Geometry: final body of the model. Coordinates: model frame, mm. Face numbers are marked on the shaded views. A direction names the side the tool comes from. Give positions to 0.01 mm unless a question says otherwise; leave off trailing zeros. Loops run counter-clockwise (first coordinate to the right, second up) from the corner with the lowest first, then second, coordinate; pieces in that order, holes last. Notation, with made-up numbers: (36.25, -30.75) -> (41.25, -30.75) arc R13 ccw to (41.25, -26.75) -> close; hole circle Ø2 at (58.25, -4.5). An arc over 180 degrees is marked (long way). One line per question, with ' | ' between items. Start each with the question number.
Item 1: Material intervals for line 1 along Y through (x, z) = (-3, 18.5); line 2 along Y through (x, z) = (-0.5, 17.5); line 3 along Z through (x, y) = (2.5, 27), sorted ascending. Write a range as [from, to].
Item 2: Pin query (flat end, axial travel): P1, Ø1.5, axis at x = 1.5, y = 40.5, coming from the -Z side; P2, Ø3, axis at x = 1, z = -6.5, coming from the +Y side; P3, Ø1.2, axis at x = -2, z = 15, coming from the +Y side; P4, Ø12, axis at y = 40, z = 13.5, coming from the +X side. Return the tip coordinate at first contact, or that it passes through.
Item 3: Section A-A on z = 9. Return loops of the section in (x, y) (3 decimals).
Item 4: Section C-C on z = 1.5. Return loops of the section in (x, y) (3 decimals).
Item 5: Section B-B on y = 24.5. Return loops of the section in (x, z) (3 decimals), then the cut area to 3 significant figures.
Item 6: Set-up query: the marked faces 1, 2 and 3. Return all of +Z, -Z, +X, -X, +Y, -Y with unobstructed straight access to the full face (end or side cutting, diameter ignored); none if empty.
Item 7: Mould query, pull axis Y, two halves, no side actions, for the marked faces 4, 5, 6 and 7. Classes: released by +Y, released by -Y, zero draft, split by the parting line, or undercut.
from build123d import *

# Parameters (mm, degrees)
F1_DEPTH = 4.445
F2_R     = 2.032
F4_DEPTH = 8.891
F5_R     = 0.762
F7_DEPTH = 8.89


# Not quite as in the source:
# - a feature names something its author has since deleted; it is built from what else it names


with BuildPart() as f1:
    # F0 (on Right) → F1 (new body, symmetric)
    with BuildSketch(Plane.YZ):
        with BuildLine():
            Line((12.7, 27.94), (0, 27.94))
            Line((0, 27.94), (0, -27.94))
            Line((0, -27.94), (12.7, -27.94))
            Line((12.7, -27.94), (12.7, -16.51))
            ThreePointArc((12.7, -16.51), (15.6757951031, -9.3257951031), (22.86, -6.35))
            Line((22.86, -6.35), (49.2345620046, -6.35))
            ThreePointArc((49.2345620046, -6.35), (52.1666656987, -5.6325187907), (54.4361774858, -3.6422103708))
            Line((54.4361774858, -3.6422103708), (69.5640047708, 17.9625660125))
            Line((69.5640047708, 17.9625660125), (59.1607738083, 25.2469867541))
            Line((59.1607738083, 25.2469867541), (48.96258477, 10.6824634067))
            ThreePointArc((48.96258477, 10.6824634067), (45.3313659105, 7.4979699349), (40.64, 6.35))
            Line((40.64, 6.35), (22.86, 6.35))
            ThreePointArc((22.86, 6.35), (15.6757951031, 9.3257951031), (12.7, 16.51))
            Line((12.7, 16.51), (12.7, 27.94))
        make_face()
    extrude(amount=F1_DEPTH, both=True)

    # F2
    f2_edges = [f1.edges().sort_by_distance(p)[0] for p in [
        (0, 12.7, 27.94),
        (0, 59.160774, 25.246987),
        (0, 69.564005, 17.962566),
        (0, 12.7, -27.94),
        (0, 0, -27.94),
        (0, 0, 27.94),
    ]]
    fillet(f2_edges, radius=F2_R)

    # F3 (on face) → F4 (cut, through all)
    with BuildSketch(Plane.YZ.offset(4.445)):
        with BuildLine():
            Line((7.62, 11.43), (7.62, 17.78))
            ThreePointArc((7.62, 17.78), (6.35, 19.05), (5.08, 17.78))
            Line((5.08, 17.78), (5.08, 13.97))
            Line((5.08, 13.97), (0, 13.97))
            Line((0, 13.97), (0, 11.43))
            Line((0, 11.43), (7.62, 11.43))
        make_face()
        with BuildLine():
            Line((7.62, -18.796), (7.62, -12.446))
            ThreePointArc((7.62, -12.446), (6.35, -11.176), (5.08, -12.446))
            Line((5.08, -12.446), (5.08, -16.256))
            Line((5.08, -16.256), (0, -16.256))
            Line((0, -16.256), (0, -18.796))
            Line((0, -18.796), (7.62, -18.796))
        make_face()
    extrude(amount=-F4_DEPTH, mode=Mode.SUBTRACT)

    # F5
    f5_edges = [f1.edges().sort_by_distance(p)[0] for p in [
        (0, 7.62, 11.43),
        (0, 0, -16.256),
        (0, 7.62, -18.796),
        (0, 0, -18.796),
        (0, 5.08, -16.256),
        (0, 5.08, 13.97),
    ]]
    fillet(f5_edges, radius=F5_R)

    # F6 (on face) → F7 (join, through all)
    with BuildSketch(Plane.YZ.offset(4.445)):
        with BuildLine():
            Line((5.08, 17.0451861632), (5.08, 15.8510145557))
            ThreePointArc((5.08, 15.8510145557), (5.2483526058, 16.4481003594), (5.08, 17.0451861632))
        make_face()
        with BuildLine():
            Line((5.08, -13.1808138368), (5.08, -14.3749854443))
            ThreePointArc((5.08, -14.3749854443), (5.2483526058, -13.7778996406), (5.08, -13.1808138368))
        make_face()
        with BuildLine():
            Line((7.62, -14.3749854443), (7.62, -13.1808138368))
            ThreePointArc((7.62, -13.1808138368), (7.4516473942, -13.7778996406), (7.62, -14.3749854443))
        make_face()
        with BuildLine():
            Line((7.62, 15.8510145557), (7.62, 17.0451861632))
            ThreePointArc((7.62, 17.0451861632), (7.4516473942, 16.4481003594), (7.62, 15.8510145557))
        make_face()
    extrude(amount=-F7_DEPTH)


solid = f1.part
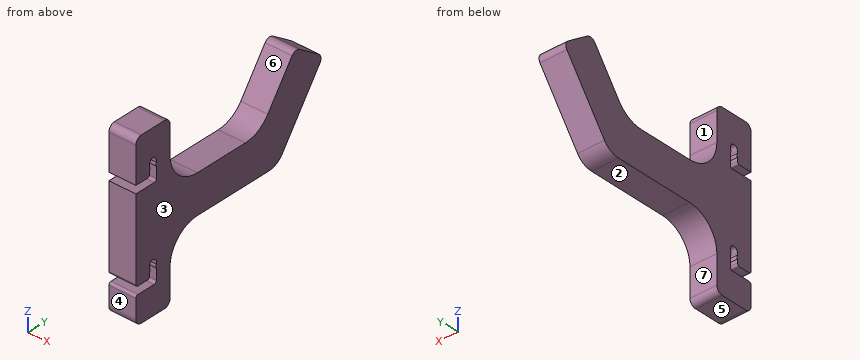
Result sheet:
1) line 1: y = [0, 5.3], [7.4, 12.7], [54.44, 68.48] | line 2: y = [0, 5.08], [7.62, 12.7], [53.74, 68.77] | line 3: z = [-6.35, 6.35]
2) P1: stops at z = -6.35 | P2: stops at y = 53.15 | P3: stops at y = 67.91 | P4: passes through
3) outline: (-4.445, 0) -> (4.445, 0) -> (4.445, 16.017) -> (-4.445, 16.017) -> close; (-4.445, 47.483) -> (4.445, 47.483) -> (4.445, 63.288) -> (-4.445, 63.288) -> close
4) outline: (-4.445, 0) -> (4.445, 0) -> (4.445, 58.037) -> (-4.445, 58.037) -> close
5) outline: (-4.445, -6.35) -> (4.445, -6.35) -> (4.445, 6.35) -> (-4.445, 6.35) -> close | area: 113 mm²
6) face 1: +Z, +X, -X | face 2: -Z, +X, -X, +Y | face 3: +Z, -Z, +X, +Y, -Y
7) face 4: released by -Y | face 5: zero draft | face 6: undercut | face 7: released by +Y
